The figure shows three views and two pictorial views of one solid part (mm, origin at its lowest corner). Answer the questions. Coordinates: 2 decimals unless noted, no trailing zeros. Write each loop counter-clockwise with the first axis right and the second up, starting at its lowest first coordinate (ties: lowest second). Pieces come first, ordered by that corner, then holes.
Item 1: Section B-B (y = 6.25) is taken. Give the vertices of the cut face in (x, z).
Item 2: Straight lines are drawn through the part: probe 1 along Y at (x, z) = (6.25, 5.5); probe 2 along Z at (x, y) = (7, 6.75); probe 3 along Z at (x, y) = (1, 4.75). For each, find the intervals that lie inside material, in ascending order.
Item 3: Section A-A (z = 6) is taken. Give the vertices of the cut face in (x, y), then the cut area to 3 significant figures.
Item 4: Section D-D (z = 18) is taken. Give the vertices of the cut face in (x, y), then the cut area to 3 significant figures.
Item 5: Each of these flat-tipped pins is pushed along its axis until it touches: P1, Ø5, axis at y = 5.5, z = 5, coming from the -X side; P2, Ø5, axis at x = 9.5, z = 6, coming from the -Y side; P3, Ø5, axis at x = 6, z = 33, coming from the -Y side; P4, Ø4, axis at x = 2, z = 32, coming from the +Y side. Where does it stop, or does it pass through?
Item 6: Determine the mould class of the marked faces 1, 2 and 3 for opening direction X: released by +X, released by -X, zero draft, split by the parting line, or undercut.
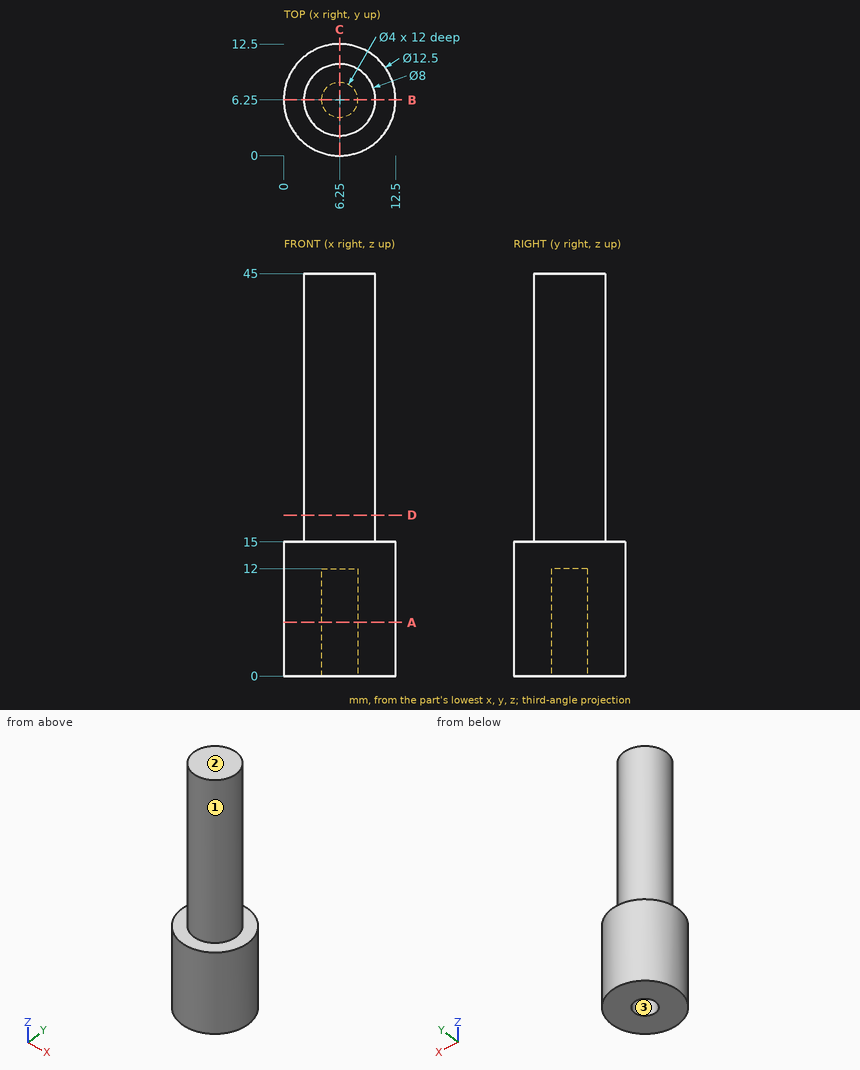
Established:
1. outline: (0, 0) - (4.25, 0) - (4.25, 12) - (8.25, 12) - (8.25, 0) - (12.5, 0) - (12.5, 15) - (10.25, 15) - (10.25, 45) - (2.25, 45) - (2.25, 15) - (0, 15) - close
2. probe 1: y = 0 to 4.25, 8.25 to 12.5
2. probe 2: z = 12 to 45
2. probe 3: z = 0 to 15
3. outline: circle Ø12.5 at (6.25, 6.25); hole circle Ø4 at (6.25, 6.25)
3. area: 110 mm2
4. outline: circle Ø8 at (6.25, 6.25)
4. area: 50.3 mm2
5. P1: stops at x = 0
5. P2: stops at y = 0.05
5. P3: stops at y = 2.25
5. P4: stops at y = 9.56
6. face 1: split by the parting line
6. face 2: zero draft
6. face 3: undercut
